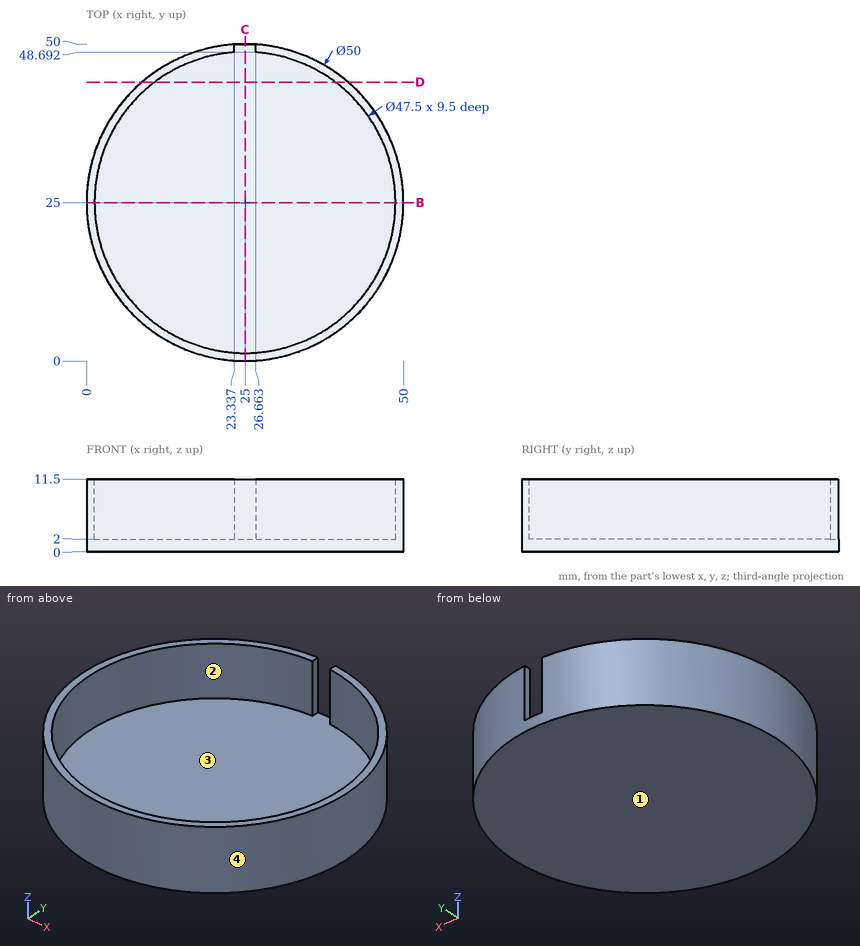
Verification items for this drawing (mm, ordinates from the low corner). Round coordinates to 2 decimals unless told otherwise and drop trailing zeros. Write each loop counter-clockwise with the first axis right and the second up, starting at its lowest first coordinate (ties: lowest second). Pieces come first, ordered by that corner, then holes. Notation, with made-up numbers: (49.5, 75.5) - (90.5, 75.5) arc R22 ccw to (90.5, 90.5) - close; hole circle Ø5 at (7.25, -39.5). An arc over 180 degrees is marked (long way). One line per item, written item: value.
1. Cross-section at D-D on y = 44. Record the boundary of the cut face in (x, z), and give its area (3 significant figures).
The answers:
outline: (8.75, 0) - (41.25, 0) - (41.25, 11.5) - (39.25, 11.5) - (39.25, 2) - (10.75, 2) - (10.75, 11.5) - (8.75, 11.5) - close
area: 103 mm^2
2. Mould release check, pull along X, two halves, no side actions. Record for the marked faces 1, 2, 3 and 4: released by +X, released by -X, zero draft, split by the parting line, or undercut.
The answers:
face 1: zero draft
face 2: undercut
face 3: undercut
face 4: split by the parting line
3. Cross-section at C-C on x = 25. Record the boundary of the cut face in (y, z), and give its area (3 significant figures).
The answers:
outline: (0, 0) - (50, 0) - (50, 2) - (1.25, 2) - (1.25, 11.5) - (0, 11.5) - close
area: 112 mm^2
4. Depth check by flat-ended pin: pin 1 Ø4 at (x, z) = (11, 2) entering from +Y; pin 2 Ø1.5 at (x, z) = (24, 4) entering from -Y; pin 3 Ø4 at (x, z) = (38, 2.5) entering from -Y. Enter the tip coordinate at first touch or a pass-through.
The answers:
pin 1: stops at y = 46.93
pin 2: stops at y = 0
pin 3: stops at y = 2.55
5. Scan lines: L1, parallel to X at y = 25, z = 4.5; L2, parallel to X at y = 17.5, z = 9 (1 decimal); L3, parallel to Z at x = 30, y = 4.5. Record each from-to range of solid material in increasing order.
The answers:
L1: x = 0 to 1.25, 48.75 to 50
L2: x = 1.2 to 2.5, 47.5 to 48.8
L3: z = 0 to 2
6. Cross-section at B-B on y = 25. Record the boundary of the cut face in (x, z), and give its area (3 significant figures).
The answers:
outline: (0, 0) - (50, 0) - (50, 11.5) - (48.75, 11.5) - (48.75, 2) - (1.25, 2) - (1.25, 11.5) - (0, 11.5) - close
area: 124 mm^2
